from build123d import *

# Parameters (mm, degrees)
F0_W     = 203.2
F0_H     = 127
F1_DEPTH = 1.27
F2_W     = 1.7448549651
F2_H     = 61.595
F2_W_2   = 46.99
F2_H_2   = 1.7448549651
F2_W_3   = 1.905
F2_W_4   = 47.1501450349
F2_H_3   = 1.905
F3_DEPTH = 50.8
F4_W     = 6.35
F4_H     = 12.7
F5_DEPTH = 25.4


with BuildPart() as f1:
    # F0 (on Top) → F1 (new body)
    with BuildSketch(Plane.XY):
        with Locations((101.6, -63.5)):
            Rectangle(F0_W, F0_H)
    extrude(amount=F1_DEPTH)

    # F2 (on Top) → F3 (join)
    with BuildSketch(Plane.XY):
        Polygon((50.8, -1.905), (48.895, -1.905), (48.895, -61.595), (1.905, -61.595), (1.905, -63.5), (50.8, -63.5), align=None)
        Polygon((1.7448549651, -1.7448549651), (1.7448549651, 0), (0, 0), (0, -61.595), (1.7448549651, -61.595), align=None)
        Polygon((52.705, -1.905), (50.8, -1.905), (50.8, -63.5), (101.6, -63.5), (101.6, -1.905), (99.695, -1.905), (99.695, -61.595), (52.705, -61.595), align=None)
        Polygon((101.6, -1.905), (101.6, -63.5), (152.4, -63.5), (152.4, -1.905), (150.495, -1.905), (150.495, -61.595), (103.505, -61.595), (103.505, -1.905), align=None)
        Polygon((152.4, -1.905), (152.4, -63.5), (201.4551450349, -63.5), (201.4551450349, -1.905), (201.295, -1.905), (201.295, -61.595), (154.305, -61.595), (154.305, -1.905), align=None)
        with Locations((202.3275725174, -32.7025)):
            Rectangle(F2_W, F2_H)
        with Locations((177.8, -0.8724274826)):
            Rectangle(F2_W_2, F2_H_2)
        Polygon((201.4551450349, -1.7448549651), (201.4551450349, -1.905), (203.2, -1.905), (203.2, 0), (201.295, 0), (201.295, -1.7448549651), align=None)
        with Locations((127, -0.8724274826)):
            Rectangle(F2_W_2, F2_H_2)
        with Locations((151.4475, -0.8724274826)):
            Rectangle(F2_W_3, F2_H_2)
        with Locations((153.3525, -0.8724274826)):
            Rectangle(F2_W_3, F2_H_2)
        with Locations((76.2, -0.8724274826)):
            Rectangle(F2_W_2, F2_H_2)
        with Locations((100.6475, -0.8724274826)):
            Rectangle(F2_W_3, F2_H_2)
        with Locations((102.5525, -0.8724274826)):
            Rectangle(F2_W_3, F2_H_2)
        with Locations((49.8475, -0.8724274826)):
            Rectangle(F2_W_3, F2_H_2)
        with Locations((51.7525, -0.8724274826)):
            Rectangle(F2_W_3, F2_H_2)
        with Locations((25.3199274826, -0.8724274826)):
            Rectangle(F2_W_4, F2_H_2)
        with Locations((0.8724274826, -62.5475)):
            Rectangle(F2_W, F2_H_3)
    extrude(amount=F3_DEPTH)

    # F4 (on face) → F5 (cut)
    with BuildSketch(Plane.XZ.offset(63.5)):
        with Locations((28.575, 7.62)):
            Rectangle(F4_W, F4_H)
        with Locations((73.025, 7.62)):
            Rectangle(F4_W, F4_H)
        with Locations((130.175, 7.62)):
            Rectangle(F4_W, F4_H)
        with Locations((174.625, 7.62)):
            Rectangle(F4_W, F4_H)
    extrude(amount=-F5_DEPTH, mode=Mode.SUBTRACT)


solid = f1.part
Geometry check sheet. Reference: the model listing, model coordinates, mm. A direction names the side the tool comes from. Coordinates: 2 decimals unless noted, no trailing zeros. Order: outer loops, then holes, each group sorted by start corner. A loop starts at its lowest first (then second) coordinate and runs counter-clockwise, first axis right, second up. Notation, with made-up numbers: (69.5, 17) - (82.5, 17) arc R23 cw to (82.5, 29) - close; hole circle Ø1 at (-17, -21). An arc over 180 degrees is marked (long way). One line per item, written item: value.
(1) Thickness scan on probe 1 along X at (y, z) = (-48, 44) (3 decimals); probe 2 along Y at (x, z) = (136.5, 28) (3 decimals); probe 3 along Z at (x, y) = (141.5, -113). Record the ranges inside material, lowest first. Write a range as from..to.
Data:
probe 1: x = 0..1.745, 48.895..52.705, 99.695..103.505, 150.495..154.305, 201.295..203.2
probe 2: y = -63.5..-61.595, -1.745..0
probe 3: z = 0..1.27
(2) Sectioned sample at D-D (x = 181.5). Enter the section's corners in (y, z) (3 decimals).
Data:
outline: (-127, 0) - (0, 0) - (0, 50.8) - (-1.745, 50.8) - (-1.745, 1.27) - (-61.595, 1.27) - (-61.595, 50.8) - (-63.5, 50.8) - (-63.5, 1.27) - (-127, 1.27) - close
(3) Release check for a two-part mould opening along X. For faces 1 (the face through (101, -63.5, 26)), 2 (the face through (102, -1.905, 26)), 3 (the face through (51, -1.905, 26)), 4 (the face through (203.2, -22, 25)) record: +X half, -X half, draft (parallel to the pull), parting line (faces both ways), or undercut.
Data:
face 1: draft
face 2: undercut
face 3: undercut
face 4: +X half
(4) Sectioned sample at A-A (x = 29). Enter the section's corners in (y, z) (3 decimals), and give its area (3 significant figures).
Data:
outline: (-127, 0) - (0, 0) - (0, 50.8) - (-1.745, 50.8) - (-1.745, 1.27) - (-127, 1.27) - close; (-63.5, 13.97) - (-61.595, 13.97) - (-61.595, 50.8) - (-63.5, 50.8) - close
area: 318 mm^2
(5) Sectioned sample at C-C (z = 38.5). Enter the section's corners in (x, y) (3 decimals), and give its area (3 significant figures).
Data:
outline: (0, -63.5) - (1.745, -63.5) - (1.745, -1.745) - (201.455, -1.745) - (201.455, -1.905) - (201.295, -1.905) - (201.295, -61.595) - (154.305, -61.595) - (154.305, -1.905) - (150.495, -1.905) - (150.495, -61.595) - (103.505, -61.595) - (103.505, -1.905) - (99.695, -1.905) - (99.695, -61.595) - (52.705, -61.595) - (52.705, -1.905) - (48.895, -1.905) - (48.895, -61.595) - (1.905, -61.595) - (1.905, -63.5) - (203.2, -63.5) - (203.2, 0) - (0, 0) - close
area: 1,640 mm^2
(6) Depth check by flat-ended pin: pin 1 Ø2 at (x, y) = (31, -101.5) entering from +Z; pin 2 Ø1.9 at (x, z) = (0.5, 20.5) entering from -Y. Enter the tip coordinate at first touch or a pass-through.
Data:
pin 1: stops at z = 1.27
pin 2: stops at y = -63.5
(7) Access from +Z, -Z, +X, -X, +Y, -Y to the whole of each face (thin tool, end or side, straight path). Record for faces 5 (the face through (0, -22, 25)), 6 (the face through (103.505, -32, 26)), 7 (the face through (1.745, -33, 26)).
Data:
face 5: +Z, -Z, -X, +Y, -Y
face 6: +Z
face 7: +Z, -Y
(8) Sectioned sample at B-B (y = -40.5). Enter the section's corners in (x, z) (3 decimals).
Data:
outline: (0, 0) - (203.2, 0) - (203.2, 50.8) - (201.295, 50.8) - (201.295, 1.27) - (154.305, 1.27) - (154.305, 50.8) - (150.495, 50.8) - (150.495, 1.27) - (103.505, 1.27) - (103.505, 50.8) - (99.695, 50.8) - (99.695, 1.27) - (52.705, 1.27) - (52.705, 50.8) - (48.895, 50.8) - (48.895, 1.27) - (1.745, 1.27) - (1.745, 50.8) - (0, 50.8) - close
